```python
from build123d import *

# Parameters (mm, degrees)
EXTRUDE_1_DEPTH     = 3
SKETCH_2_W          = 25
SKETCH_2_H          = 8
EXTRUDE_2_DEPTH     = 3
SKETCH_3_R          = 1.25
CUT_EXTRUDE_1_DEPTH = 51.635955605
SKETCH_3_3_R        = 2
CUT_EXTRUDE_2_DEPTH = 1.5
SKETCH_4_R          = 0.6
CUT_EXTRUDE_3_DEPTH = 51.635955605
SKETCH_4_3_R        = 1
CUT_EXTRUDE_4_DEPTH = 1.5
SKETCH_5_W          = 3
SKETCH_5_H          = 0.2
CUT_EXTRUDE_5_DEPTH = 31.170349683
SKETCH_6_R          = 0.6
CUT_EXTRUDE_6_DEPTH = 31.170349683
SKETCH_6_3_R        = 1
CUT_EXTRUDE_7_DEPTH = 1.5
SKETCH_7_R          = 0.35
CUT_EXTRUDE_8_DEPTH = 3
SKETCH_8_R          = 4
SKETCH_8_R_2        = 1
CUT_EXTRUDE_9_DEPTH = 31.170349683


with BuildPart() as part:
    # Sketch 1 → Extrude 1 (new body)
    with BuildSketch(Plane(origin=(0, 0, 0), x_dir=(1, 0, 0), z_dir=(0, 1, 0))):
        Polygon((-22.5, 11), (-22.5, -11), (22.5, -11), (22.5, 14), (-19.5, 14), (-19.5, 11), align=None)
    extrude(amount=EXTRUDE_1_DEPTH)

    # Sketch 2 → Extrude 2 (add)
    with BuildSketch(Plane(origin=(22.5, 0, 0), x_dir=(0, 0, -1), z_dir=(1, 0, 0))):
        with Locations((1.5, 4)):
            Rectangle(SKETCH_2_W, SKETCH_2_H)
    extrude(amount=EXTRUDE_2_DEPTH)

    # Sketch 3 → Cut-Extrude 1 (cut, through all)
    with BuildSketch(Plane(origin=(25.5, 0, 0), x_dir=(0, 0, -1), z_dir=(1, 0, 0))):
        with Locations((5.375, 5.500000041)):
            Circle(SKETCH_3_R)
        with Locations((-5.875, 5.500000041)):
            Circle(SKETCH_3_R)
    extrude(amount=-CUT_EXTRUDE_1_DEPTH, mode=Mode.SUBTRACT)

    # Sketch 3_3 → Cut-Extrude 2 (cut)
    with BuildSketch(Plane(origin=(25.5, 0, 0), x_dir=(0, 0, -1), z_dir=(1, 0, 0))):
        with Locations((5.375, 5.500000041)):
            Circle(SKETCH_3_3_R)
        with Locations((-5.875, 5.500000041)):
            Circle(SKETCH_3_3_R)
    extrude(amount=-CUT_EXTRUDE_2_DEPTH, mode=Mode.SUBTRACT)

    # Sketch 4 → Cut-Extrude 3 (cut, through all)
    with BuildSketch(Plane(origin=(25.5, 0, 0), x_dir=(0, 0, -1), z_dir=(1, 0, 0))):
        with Locations((12.5, 5.5)):
            Circle(SKETCH_4_R)
    extrude(amount=-CUT_EXTRUDE_3_DEPTH, mode=Mode.SUBTRACT)

    # Sketch 4_3 → Cut-Extrude 4 (cut)
    with BuildSketch(Plane(origin=(25.5, 0, 0), x_dir=(0, 0, -1), z_dir=(1, 0, 0))):
        with Locations((12.5, 5.5)):
            Circle(SKETCH_4_3_R)
    extrude(amount=-CUT_EXTRUDE_4_DEPTH, mode=Mode.SUBTRACT)

    # Sketch 5 → Cut-Extrude 5 (cut, through all)
    with BuildSketch(Plane.XZ):
        with Locations((-21, -10.9)):
            Rectangle(SKETCH_5_W, SKETCH_5_H)
    extrude(amount=-CUT_EXTRUDE_5_DEPTH, mode=Mode.SUBTRACT)

    # Sketch 6 → Cut-Extrude 6 (cut, through all)
    with BuildSketch(Plane.XZ):
        with Locations(Location((-10.5, -12.5, 0), (0, 0, 270))):
            Circle(SKETCH_6_R)
        with Locations(Location((13.5, -12.5, 0), (0, 0, 270))):
            Circle(SKETCH_6_R)
    extrude(amount=-CUT_EXTRUDE_6_DEPTH, mode=Mode.SUBTRACT)

    # Sketch 6_3 → Cut-Extrude 7 (cut)
    with BuildSketch(Plane.XZ):
        with Locations(Location((-10.5, -12.5, 0), (0, 0, 270))):
            Circle(SKETCH_6_3_R)
        with Locations(Location((13.5, -12.5, 0), (0, 0, 270))):
            Circle(SKETCH_6_3_R)
    extrude(amount=-CUT_EXTRUDE_7_DEPTH, mode=Mode.SUBTRACT)

    # Sketch 7 → Cut-Extrude 8 (cut)
    with BuildSketch(Plane.XZ):
        with Locations(Location((21, 4.75, 0), (0, 0, 270))):
            Circle(SKETCH_7_R)
        with Locations(Location((21, -7.75, 0), (0, 0, 270))):
            Circle(SKETCH_7_R)
    extrude(amount=-CUT_EXTRUDE_8_DEPTH, mode=Mode.SUBTRACT)

    # Sketch 8 → Cut-Extrude 9 (cut, through all)
    with BuildSketch(Plane.XZ):
        with Locations(Location((-5.5, 3.5, 0), (0, 0, 270))):
            Circle(SKETCH_8_R)
        with Locations(Location((15.5, 9.5, 0), (0, 0, 270))):
            Circle(SKETCH_8_R_2)
        with Locations(Location((15.5, 5.5, 0), (0, 0, 270))):
            Circle(SKETCH_8_R_2)
        with Locations(Location((15.5, 1.5, 0), (0, 0, 270))):
            Circle(SKETCH_8_R_2)
        with Locations(Location((15.5, -2.5, 0), (0, 0, 270))):
            Circle(SKETCH_8_R_2)
    extrude(amount=-CUT_EXTRUDE_9_DEPTH, mode=Mode.SUBTRACT)


solid = part.part
```
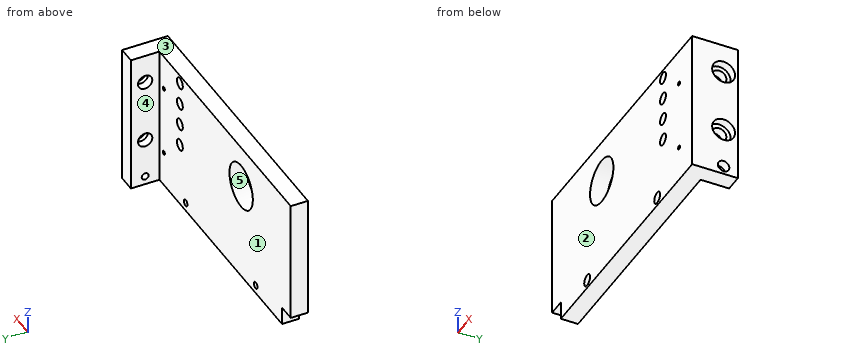
Could you check a few things on this model? Use its own coordinates, in mm. Face numbers are marked on the shaded views. A direction names the side the tool comes from. Round coordinates to 2 decimals unless told otherwise and drop trailing zeros. Write each loop counter-clockwise with the first axis right and the second up, starting at its lowest first coordinate (ties: lowest second). Pieces come first, ordered by that corner, then holes.
(1) Suppose I cut it at A-A on x = 13.5. Write out the boundary of the cut face in (y, z).
Findings below:
outline: (0, -14) - (3, -14) - (3, -13.1) - (1.5, -13.1) - (1.5, -13.5) - (0, -13.5) - close; (0, -11.5) - (1.5, -11.5) - (1.5, -11.9) - (3, -11.9) - (3, 11) - (0, 11) - close
(2) Which directions (+Z, -Z, +X, -X, +Y, -Y) give clear straight access to the entire face, cutting with the end or side of a thin tool? Please do the marked faces 1 and 2.
Findings below:
face 1: +Z, -Z, -X, +Y
face 2: +Z, -Z, +X, -X, -Y
(3) Thinking about a two-plate mould opening in Z: for the marked faces 3, 4 and 5, which applies, +Z half, -Z half, draft (parallel to the pull), parting line (faces both ways), or undercut?
Findings below:
face 3: +Z half
face 4: draft
face 5: undercut
(4) Suppose I cut it at C-C on z = 3. Write out the boundary of the cut face in (x, y), and give its area (3 significant figures).
Findings below:
outline: (-22.5, 0) - (-9.47, 0) - (-9.47, 3) - (-22.5, 3) - close; (-1.53, 0) - (25.5, 0) - (25.5, 8) - (22.5, 8) - (22.5, 3) - (-1.53, 3) - close
area: 135 mm2
(5) Suppose I cut it at B-B on y = 5.5. Write out the boundary of the cut face in (x, z) (3 decimals).
Findings below:
outline: (22.5, -14) - (25.5, -14) - (25.5, -13.5) - (24, -13.5) - (24, -13.1) - (22.5, -13.1) - close; (22.5, -11.9) - (24, -11.9) - (24, -11.5) - (25.5, -11.5) - (25.5, -7.375) - (24, -7.375) - (24, -6.625) - (22.5, -6.625) - close; (22.5, -4.125) - (24, -4.125) - (24, -3.375) - (25.5, -3.375) - (25.5, 3.875) - (24, 3.875) - (24, 4.625) - (22.5, 4.625) - close; (22.5, 7.125) - (24, 7.125) - (24, 7.875) - (25.5, 7.875) - (25.5, 11) - (22.5, 11) - close
(6) Suppose I cut it at D-D on x = -6.5. Write out the boundary of the cut face in (y, z).
Findings below:
outline: (0, -14) - (3, -14) - (3, -0.37) - (0, -0.37) - close; (0, 7.37) - (3, 7.37) - (3, 11) - (0, 11) - close
(7) If I drill on probe 1 along X at (y, z) = (2.5, -12.5); probe 2 along Z at (x, y) = (21, 0.6); probe 3 along X at (y, z) = (0.9, 1.5), over which ranges is the centre line in solid material (lowest first)?
Findings below:
probe 1: x = -19.5 to -11.1, -9.9 to 12.9, 14.1 to 25.5
probe 2: z = -14 to -8.1, -7.4 to 4.4, 5.1 to 11
probe 3: x = -22.5 to -8.96, -2.04 to 14.5, 16.5 to 25.5
(8) For pin 1 (2.5 mm diameter, centred on x = 15.5, z = 1.5, fed in from +Y); pin 2 (3 mm diameter, centred on y = 5.5, z = 5.875, fed in from +X); pin 3 (0.6 mm diameter, centred on x = 14, z = -12.5, fed in from -Y); pin 4 (2 mm diameter, centred on x = 16.5, y = 5, fed in from -Z), each with a flat end and sliding along its axis, tell me the tip position at first contact or that it passes through.
Findings below:
pin 1: stops at y = 3
pin 2: stops at x = 24
pin 3: stops at y = 1.5
pin 4: passes through
